from build123d import *

# Parameters (mm, degrees)
SKETCH_1_R      = 1.55
EXTRUDE_1_DEPTH = 2


with BuildPart() as part:
    # 草图1 → 凸台-拉伸1 (new body)
    with BuildSketch(Plane.XY):
        with BuildLine():
            Line((-53, 72.523086953), (-53, 52.405955819))
            Line((-53, 52.405955819), (-49.8, 52.405955819))
            Line((-49.8, 52.405955819), (-49.8, 45.507725731))
            Line((-49.8, 45.507725731), (-53, 45.507725731))
            Line((-53, 45.507725731), (-53, 20.011565656))
            Line((-53, 20.011565656), (-40, 20.011565656))
            ThreePointArc((-40, 20.011565656), (-38.585786438, 19.425779218), (-38, 18.011565656))
            Line((-38, 18.011565656), (-38, -21.289037005))
            ThreePointArc((-38, -21.289037005), (-38.585786438, -22.703250568), (-40, -23.289037005))
            Line((-40, -23.289037005), (-53, -23.289037005))
            Line((-53, -23.289037005), (-53, -26.067193504))
            Line((-53, -26.067193504), (-49.8, -26.067193504))
            Line((-49.8, -26.067193504), (-49.8, -32.930143701))
            Line((-49.8, -32.930143701), (-53, -32.930143701))
            Line((-53, -32.930143701), (-53, -61.384473154))
            Line((-53, -61.384473154), (53, -61.384473154))
            Line((53, -61.384473154), (53, -32.930143701))
            Line((53, -32.930143701), (49.8, -32.930143701))
            Line((49.8, -32.930143701), (49.8, -26.067193504))
            Line((49.8, -26.067193504), (53, -26.067193504))
            Line((53, -26.067193504), (53, -23.289037005))
            Line((53, -23.289037005), (40, -23.289037005))
            ThreePointArc((40, -23.289037005), (38.585786438, -22.703250568), (38, -21.289037005))
            Line((38, -21.289037005), (38, 18.011565656))
            ThreePointArc((38, 18.011565656), (38.585786438, 19.425779218), (40, 20.011565656))
            Line((40, 20.011565656), (53, 20.011565656))
            Line((53, 20.011565656), (53, 45.507725731))
            Line((53, 45.507725731), (49.8, 45.507725731))
            Line((49.8, 45.507725731), (49.8, 52.405955819))
            Line((49.8, 52.405955819), (53, 52.405955819))
            Line((53, 52.405955819), (53, 67.484473154))
            Line((53, 67.484473154), (53, 72.523086953))
            Line((53, 72.523086953), (49.8, 72.523086953))
            Line((49.8, 72.523086953), (49.8, 79.540910094))
            Line((49.8, 79.540910094), (53, 79.540910094))
            Line((53, 79.540910094), (53, 107.384473154))
            Line((53, 107.384473154), (-53, 107.384473154))
            Line((-53, 107.384473154), (-53, 79.540910094))
            Line((-53, 79.540910094), (-49.8, 79.540910094))
            Line((-49.8, 79.540910094), (-49.8, 72.523086953))
            Line((-49.8, 72.523086953), (-53, 72.523086953))
        make_face()
        with Locations((-42.5, 63.5)):
            Circle(SKETCH_1_R, mode=Mode.SUBTRACT)
        with Locations((32.5, 63.515526846)):
            Circle(SKETCH_1_R, mode=Mode.SUBTRACT)
        with Locations((-42.5, 41.5)):
            Circle(SKETCH_1_R, mode=Mode.SUBTRACT)
        with Locations((32.5, 41.515526846)):
            Circle(SKETCH_1_R, mode=Mode.SUBTRACT)
        with Locations((-46, -29.484473154)):
            Circle(SKETCH_1_R, mode=Mode.SUBTRACT)
        with Locations((46, -29.484473154)):
            Circle(SKETCH_1_R, mode=Mode.SUBTRACT)
        with BuildLine():
            Line((-16.369193533, 77.65782048), (23.228994882, 77.65782048))
            ThreePointArc((23.228994882, 77.65782048), (24.643208444, 77.072034042), (25.228994882, 75.65782048))
            Line((25.228994882, 75.65782048), (25.228994882, 32.660489145))
            ThreePointArc((25.228994882, 32.660489145), (24.643208444, 31.246275583), (23.228994882, 30.660489145))
            Line((23.228994882, 30.660489145), (-16.369193533, 30.660489145))
            ThreePointArc((-16.369193533, 30.660489145), (-17.783407096, 31.246275583), (-18.369193533, 32.660489145))
            Line((-18.369193533, 32.660489145), (-18.369193533, 75.65782048))
            ThreePointArc((-18.369193533, 75.65782048), (-17.783407096, 77.072034042), (-16.369193533, 77.65782048))
        make_face(mode=Mode.SUBTRACT)
    extrude(amount=EXTRUDE_1_DEPTH)


solid = part.part
Could you check a few things on this model? Use its own coordinates, in mm. Give positions to 0.01 mm unless a question says otherwise; leave off trailing zeros. Order: outer loops, then holes, each group sorted by start corner. A loop starts at its lowest first (then second) coordinate and runs counter-clockwise, first axis right, second up.
Item 1: I need wall thicknesses on line 1 (Y direction, x = -42.5, z = 1); line 2 (Y direction, x = 32.5, z = 0.7); line 3 (Y direction, x = 46, z = 0.9). Which ranges of each line are inside material? Lowest first, please.
Item 2: I'm going to push flat-ended pins straight in: pin 1 (1.9 mm diameter, centred on x = 32.5, y = 63.52, fed in from -Z) (3 decimals); pin 2 (1 mm diameter, centred on y = -10, z = 1, fed in from +X). Where does each tip first touch, or does it pass through?
Item 3: If we mould it in two halves opening along X, with no side actions, what happens to faces 1 (the face through (33.215, 62.14, 0.986)), 2 (the face through (33.333, 42.822, 0.986)), 3 (the face through (-1, 24, 2))? For each: pulls with the +X half, pulls with the -X half, needs draft (parallel to the pull), parting line crosses it, or undercut.
Item 4: If we section it at A-A, the plane z = 0.95: Count the separate pieces of the cut face and the enclosed holes in it, plus the area to 3 significant figures.
Item 5: If we section it at B-B, the plane y = -11.5: Write out the boundary of the cut face in (x, z), plus the area to 3 significant figures.
Values:
1. line 1: y = -61.38 to -23.29, 20.01 to 39.95, 43.05 to 61.95, 65.05 to 107.38
1. line 2: y = -61.38 to 39.97, 43.07 to 61.97, 65.07 to 107.38
1. line 3: y = -61.38 to -31.03, -27.93 to -23.29, 20.01 to 107.38
2. pin 1: passes through
2. pin 2: stops at x = 38
3. face 1: undercut
3. face 2: undercut
3. face 3: needs draft
4. separate pieces: 1
4. enclosed holes: 7
4. area: 14,400 mm2
5. outline: (-38, 0) - (38, 0) - (38, 2) - (-38, 2) - close
5. area: 152 mm2
